```python
from build123d import *

# Parameters (mm, degrees)
SKETCH1_R           = 4
BOSS_EXTRUDE1_DEPTH = 50
BOSS_EXTRUDE2_DEPTH = 10
SKETCH3_R           = 5
CUT_EXTRUDE1_DEPTH  = 21
SKETCH4_W           = 10
SKETCH4_H           = 22.5
CUT_EXTRUDE2_DEPTH  = 16
BOSS_EXTRUDE3_DEPTH = 5
SKETCH6_R           = 5
CUT_EXTRUDE3_DEPTH  = 20


with BuildPart() as part:
    # Sketch1 → Boss-Extrude1 (new body, symmetric)
    with BuildSketch(Plane(origin=(0, 0, 0), x_dir=(1, 0, 0), z_dir=(0, 1, 0))):
        Circle(SKETCH1_R)
    extrude(amount=BOSS_EXTRUDE1_DEPTH, both=True)

    # Sketch2 → Boss-Extrude2 (add, symmetric)
    with BuildSketch(Plane(origin=(0, 0, 0), x_dir=(0, 0, -1), z_dir=(1, 0, 0))):
        with BuildLine():
            Line((0, 50), (7.5, 50))
            Line((7.5, 50), (7.5, 70))
            ThreePointArc((7.5, 70), (0, 77.5), (-7.5, 70))
            Line((-7.5, 70), (-7.5, 50))
            Line((-7.5, 50), (0, 50))
        make_face()
    extrude(amount=BOSS_EXTRUDE2_DEPTH, both=True)

    # Sketch3 → Cut-Extrude1 (cut, through all)
    with BuildSketch(Plane(origin=(10, 0, 0), x_dir=(0, 0, -1), z_dir=(1, 0, 0))):
        with Locations((0, 70)):
            Circle(SKETCH3_R)
    extrude(amount=-CUT_EXTRUDE1_DEPTH, mode=Mode.SUBTRACT)

    # Sketch4 → Cut-Extrude2 (cut, through all)
    with BuildSketch(Plane.XY.offset(7.5)):
        with Locations((0, 66.25)):
            Rectangle(SKETCH4_W, SKETCH4_H)
    extrude(amount=-CUT_EXTRUDE2_DEPTH, mode=Mode.SUBTRACT)

    # Sketch5 → Boss-Extrude3 (add, symmetric)
    with BuildSketch(Plane(origin=(0, 0, 0), x_dir=(0, 0, -1), z_dir=(1, 0, 0))):
        with BuildLine():
            Line((-7.5, -50), (7.5, -50))
            Line((7.5, -50), (7.5, -70))
            ThreePointArc((7.5, -70), (0, -77.5), (-7.5, -70))
            Line((-7.5, -70), (-7.5, -50))
        make_face()
    extrude(amount=BOSS_EXTRUDE3_DEPTH, both=True)

    # Sketch6 → Cut-Extrude3 (cut)
    with BuildSketch(Plane(origin=(5, 0, 0), x_dir=(0, 0, -1), z_dir=(1, 0, 0))):
        with Locations((0, -70)):
            Circle(SKETCH6_R)
    extrude(amount=-CUT_EXTRUDE3_DEPTH, mode=Mode.SUBTRACT)


solid = part.part
```
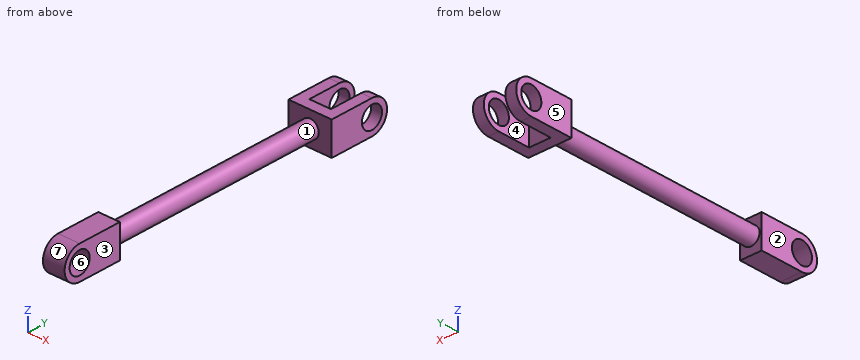
Input: part model. Units: mm. Frame: model coordinates. Face numbers are marked on the shaded views. A direction names the side the tool comes from. Coordinates: 2 decimals unless noted, no trailing zeros. Order: outer loops, then holes, each group sorted by start corner. A loop starts at its lowest first (then second) coordinate and runs counter-clockwise, first axis right, second up. Notation, with made-up numbers: (3, -33) - (61, -33) arc R17 cw to (61, -18) - close; hole circle Ø1 at (18.5, 85). An arc over 180 degrees is marked (long way). Return JSON: item names as keys, results as strings.
Q1. Ray query, probe 1 along Y at (x, z) = (-8.65, 0); probe 2 along Y at (x, z) = (3.5, -3.5); probe 3 along Y at (x, z) = (3.5, -2.25). Return the intervals inside material, ascending.
The answers:
{"probe 1": "y = 50 to 65, 75 to 77.5", "probe 2": "y = -76.63 to -73.57, -66.43 to -50, 50 to 55", "probe 3": "y = -77.15 to -74.47, -65.53 to -50, 50 to 55"}
Q2. Cut plane C-C (x = 0). Return loops of the section in (y, z).
The answers:
{"outline": "(-70, -7.5) - (-50, -7.5) - (-50, -4) - (50, -4) - (50, -7.5) - (55, -7.5) - (55, 7.5) - (50, 7.5) - (50, 4) - (-50, 4) - (-50, 7.5) - (-70, 7.5) arc R7.5 ccw to start; hole circle Ø10 at (-70, 0)"}
Q3. Draft query along Y for the marked faces 5, 6 and 7. Return one class per face: +Y half, -Y half, draft (parallel to the pull), parting line (faces both ways), or undercut.
The answers:
{"face 5": "draft", "face 6": "undercut", "face 7": "-Y half"}
Q4. First-contact query: pin 1 (4.5 mm diameter, centred on y = -59.5, z = 2.5, fed in from -X); pin 2 (7.5 mm diameter, centred on y = -60, z = 0, fed in from +X); pin 3 (1.5 mm diameter, centred on x = -6, z = -4, fed in from -Y); pin 4 (6 mm diameter, centred on y = -70, z = 0, fed in from +X). Flat tips, straight axial feed; report the tip coordinate or a pass-through.
The answers:
{"pin 1": "stops at x = -5", "pin 2": "stops at x = 5", "pin 3": "stops at y = 50", "pin 4": "passes through"}
Q5. Access query for the marked faces 1, 2, 3 and 4. Directions: +Z, -Z, +X, -X, +Y, -Y. A direction counts if a zero-diameter tool reaches every point of the face in a straight line with its end or side. Return the directions, or none.
The answers:
{"face 1": "none", "face 2": "+Z, -Z, -X, -Y", "face 3": "+Z, -Z, +X, -Y", "face 4": "+Z, -Z, +Y"}
Q6. Cut plane B-B (x = 6.75). Return loops of the section in (y, z), then the cut area to 3 significant figures.
The answers:
{"outline": "(50, -7.5) - (70, -7.5) arc R7.5 ccw to (70, 7.5) - (50, 7.5) - close; hole circle Ø10 at (70, 0)", "area": "310 mm2"}
Q7. Cut plane D-D (y = 19). Return loops of the section in (x, z), then the cut area to 3 significant figures.
The answers:
{"outline": "circle Ø8 at (0, 0)", "area": "50.3 mm2"}
Q8. Cut plane A-A (y = 67). Return loops of the section in (x, z).
The answers:
{"outline": "(-10, -7.5) - (-5, -7.5) - (-5, -4) - (-10, -4) - close; (-10, 4) - (-5, 4) - (-5, 7.5) - (-10, 7.5) - close; (5, -7.5) - (10, -7.5) - (10, -4) - (5, -4) - close; (5, 4) - (10, 4) - (10, 7.5) - (5, 7.5) - close"}
